```python
from build123d import *

# Parameters (mm, degrees)
SKETCH2_W           = 10
SKETCH2_H           = 10
BOSS_EXTRUDE1_DEPTH = 5
SKETCH4_W           = 15
SKETCH4_H           = 27.94
BOSS_EXTRUDE4_DEPTH = 4
SKETCH5_W           = 2.25448465
SKETCH5_H           = 27.94
BOSS_EXTRUDE5_DEPTH = 4
SKETCH6_R           = 1.5
CUT_EXTRUDE1_DEPTH  = 40
SKETCH7_R           = 3.5
BOSS_EXTRUDE6_DEPTH = 8
SKETCH8_W           = 15
SKETCH8_H           = 27.94
CUT_EXTRUDE2_DEPTH  = 8


with BuildPart() as part:
    # Sketch2 → Boss-Extrude1 (new body)
    with BuildSketch(Plane.XY):
        with Locations((5, 5)):
            Rectangle(SKETCH2_W, SKETCH2_H)
    extrude(amount=BOSS_EXTRUDE1_DEPTH)

    # Sketch4 → Boss-Extrude4 (add)
    with BuildSketch(Plane.XY.offset(5)):
        with Locations((7.5, 5)):
            Rectangle(SKETCH4_W, SKETCH4_H)
    extrude(amount=BOSS_EXTRUDE4_DEPTH)

    # Sketch5 → Boss-Extrude5 (add)
    with BuildSketch(Plane.XY.offset(9)):
        with Locations((13.872757675, 5)):
            Rectangle(SKETCH5_W, SKETCH5_H)
    extrude(amount=BOSS_EXTRUDE5_DEPTH)

    # Sketch6 → Cut-Extrude1 (cut)
    with BuildSketch(Plane.ZY.offset(-12.74551535)):
        with Locations((11.286, 16.64426)):
            Circle(SKETCH6_R)
        with Locations((11.286, -6.645)):
            Circle(SKETCH6_R)
    extrude(amount=-CUT_EXTRUDE1_DEPTH, mode=Mode.SUBTRACT)

    # Sketch7 → Boss-Extrude6 (add)
    with BuildSketch(Plane(origin=(0, 0, 0), x_dir=(-1, 0, 0), z_dir=(0, 0, -1))):
        with Locations((-5, 5)):
            Circle(SKETCH7_R)
    extrude(amount=BOSS_EXTRUDE6_DEPTH)

    # Sketch8 → Cut-Extrude2 (cut)
    with BuildSketch(Plane.XY.offset(13)):
        with Locations((7.5, 5)):
            Rectangle(SKETCH8_W, SKETCH8_H)
    extrude(amount=-CUT_EXTRUDE2_DEPTH, mode=Mode.SUBTRACT)


solid = part.part
```
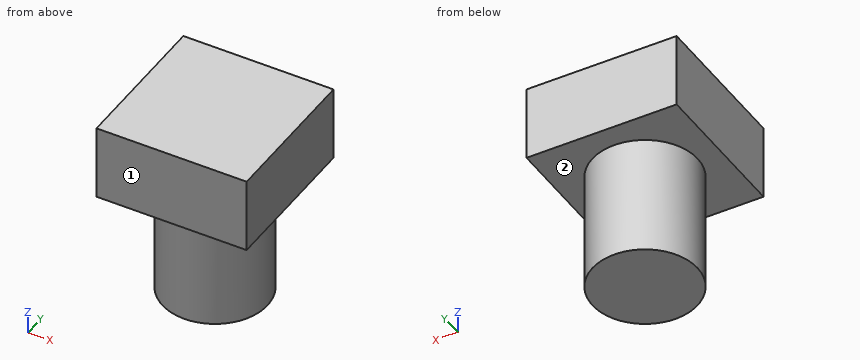
The model under review builds one solid part; all positions refer to its coordinate system, in mm. Face numbers are marked on the shaded views. A direction names the side the tool comes from. Give positions to 0.01 mm unless a question says otherwise; leave off trailing zeros. Write each loop counter-clockwise with the first axis right and the second up, starting at its lowest first coordinate (ties: lowest second). Pieces come first, ordered by that corner, then holes. Notation, with made-up numbers: M 2.5,44 L 21.5,44 A27 ccw 21.5,72 Z; hole C 41.25,-5.5 d2. An arc over 180 degrees is marked long. Answer in a Markdown table with one row per item.
Item 1: Add section A-A on y = 5. Give the boundary of the cut face in (x, z), plus the area to 3 significant figures.
Check sheet entries:
| item | result |
|---|---|
| outline | M 0,0 L 1.5,0 L 1.5,-8 L 8.5,-8 L 8.5,0 L 10,0 L 10,5 L 0,5 Z |
| area | 106 mm2 |
Item 2: For P1, Ø1, axis at y = 8.5, z = -1.5, coming from the -X side; P2, Ø3, axis at x = 4, z = -0.5, coming from the +Y side; P3, Ø1, axis at x = 6.5, z = -4, coming from the -Y side, all flat-tipped, find the tip position at first contact; note any pin that passes through.
Check sheet entries:
| item | result |
|---|---|
| P1 | x = 3.2 |
| P2 | y = 10 |
| P3 | y = 1.65 |
Item 3: Add section B-B on x = 5.5. Give the boundary of the cut face in (y, z).
Check sheet entries:
| item | result |
|---|---|
| outline | M 0,0 L 1.54,0 L 1.54,-8 L 8.46,-8 L 8.46,0 L 10,0 L 10,5 L 0,5 Z |
Item 4: Add section C-C on z = -5.5. Give the boundary of the cut face in (x, y), plus the area to 3 significant figures.
Check sheet entries:
| item | result |
|---|---|
| outline | C 5,5 d7 |
| area | 38.5 mm2 |
Item 5: For line 1 along Z through (x, y) = (6.5, 1.75); line 2 along X through (y, z) = (7.75, -4.75); line 3 along Y through (x, z) = (5.5, -5.75), list the stretches that pass through material, from the lowest coordinate up.
Check sheet entries:
| item | result |
|---|---|
| line 1 | 0 to 5 |
| line 2 | 2.83 to 7.17 |
| line 3 | 1.54 to 8.46 |
Item 6: Add section D-D on y = 1. Give the boundary of the cut face in (x, z), plus the area to 3 significant figures.
Check sheet entries:
| item | result |
|---|---|
| outline | M 0,0 L 10,0 L 10,5 L 0,5 Z |
| area | 50.0 mm2 |
Item 7: Tool access review of the marked faces 1 and 2: name each direction out of +Z, -Z, +X, -X, +Y, -Y from which nothing blocks a thin tool from reaching the whole face with its end or side.
Check sheet entries:
| item | result |
|---|---|
| face 1 | +Z, -Z, +X, -X, -Y |
| face 2 | -Z |
